Verification items for the finished model (mm, model axes). A direction names the side the tool comes from. Round coordinates to 2 decimals unless told otherwise and drop trailing zeros. Order: outer loops, then holes, each group sorted by start corner. A loop starts at its lowest first (then second) coordinate and runs counter-clockwise, first axis right, second up. Notation, with made-up numbers: (-6.75, 65.5) -> (51.25, 65.5) arc R27 ccw to (51.25, 104.5) -> close; hole circle Ø5 at (-40, 86). An arc over 180 degrees is marked (long way). Return JSON: item names as keys, results as strings. Group by question number.
1) Scan lines: L1, parallel to X at y = 0.35, z = -7; L2, parallel to X at y = 1.25, z = 11; L3, parallel to Z at x = -37, y = 2.1. Record each from-to range of solid material in increasing order.
2) Depth check by flat-ended pin: pin 1 (1.5 mm diameter, centred on x = 78, y = 1.5, fed in from -Z); pin 2 (8 mm diameter, centred on x = 4, z = -8, fed in from +Y). Enter the tip coordinate at first touch or a pass-through.
3) Section check D-D on z = 22.5. Enter the section's corners in (x, y), plus the area to 3 significant figures.
4) Section check B-B on x = -63. Enter the section's corners in (y, z).
5) Section check C-C on z = 0. State how many separate pieces and enclosed holes the cut face has, plus the area to 3 significant figures.
6) Tool access check on faces 4 (the flat face through (-18, 2, -25)), 5 (the flat face through (78, 2, -7.5)), 6 (the flat face through (-79, 2, -17.5)), 7 (the flat face through (18, 2, 25)). Record the directions out of +Z, -Z, +X, -X, +Y, -Y that give a thin tool (end or side, any length) a straight path to the whole face; none if there is none.
7) Draft check along Z on faces 1 (the flat face through (45, 2, -26)), 2 (the flat face through (-63, 2, -25)), 3 (the flat face through (-50, 2, 5.75)). Enter one of: pulls with the +Z half, pulls with the -Z half, needs draft (parallel to the pull), parting line crosses it, or undercut.
8) Section check A-A on z = 10. Enter the section's corners in (x, y).
```python
from build123d import *

# Parameters (mm, degrees)
SKETCH3_W           = 160
SKETCH3_H           = 56
BOSS_EXTRUDE1_DEPTH = 3
SKETCH4_W           = 3
SKETCH4_H           = 10
SKETCH4_W_2         = 35
SKETCH4_H_2         = 3
CUT_EXTRUDE1_DEPTH  = 85.811555816
SKETCH5_R           = 1.6
SKETCH5_R_2         = 1.5
SKETCH5_W           = 34.5
SKETCH5_H           = 24.5
SKETCH5_W_2         = 11
SKETCH5_H_2         = 30
SKETCH5_W_3         = 12.5
SKETCH5_H_3         = 11.5
CUT_EXTRUDE2_DEPTH  = 85.811555816


with BuildPart() as part:
    # Sketch3 → Boss-Extrude1 (new body)
    with BuildSketch(Plane(origin=(0, 0, 0), x_dir=(1, 0, 0), z_dir=(0, 1, 0))):
        Rectangle(SKETCH3_W, SKETCH3_H)
    extrude(amount=BOSS_EXTRUDE1_DEPTH)

    # Sketch4 → Cut-Extrude1 (cut, through all)
    with BuildSketch(Plane(origin=(0, 3, 0), x_dir=(1, 0, 0), z_dir=(0, 1, 0))):
        with Locations((-78.5, 12.5)):
            Rectangle(SKETCH4_W, SKETCH4_H)
        Polygon((-35, 28), (-35, 25), (-1.5, 25), (-1.5, 20.5), (-3, 20.5), (-3, 18), (3, 18), (3, 20.5), (1.5, 20.5), (1.5, 25), (35, 25), (35, 28), align=None)
        with Locations((-62.5, 26.5)):
            Rectangle(SKETCH4_W_2, SKETCH4_H_2)
        with Locations((62.5, 26.5)):
            Rectangle(SKETCH4_W_2, SKETCH4_H_2)
        with Locations((78.5, 12.5)):
            Rectangle(SKETCH4_W, SKETCH4_H)
        with Locations((78.5, -12.5)):
            Rectangle(SKETCH4_W, SKETCH4_H)
        with Locations((62.5, -26.5)):
            Rectangle(SKETCH4_W_2, SKETCH4_H_2)
        Polygon((35, -28), (-35, -28), (-35, -25), (-1.5, -25), (-1.5, -20.5), (-3, -20.5), (-3, -18), (3, -18), (3, -20.5), (1.5, -20.5), (1.5, -25), (35, -25), align=None)
        with Locations((-62.5, -26.5)):
            Rectangle(SKETCH4_W_2, SKETCH4_H_2)
        with Locations((-78.5, -12.5)):
            Rectangle(SKETCH4_W, SKETCH4_H)
    extrude(amount=-CUT_EXTRUDE1_DEPTH, mode=Mode.SUBTRACT)

    # Sketch5 → Cut-Extrude2 (cut, through all)
    with BuildSketch(Plane(origin=(0, 3, 0), x_dir=(1, 0, 0), z_dir=(0, 1, 0))):
        with Locations(Location((-21.5, 0, 0), (0, 0, 270))):
            Circle(SKETCH5_R)
        with Locations(Location((21.5, 0, 0), (0, 0, 90))):
            Circle(SKETCH5_R)
        with Locations(Location((-63, 0, 0), (0, 0, 270))):
            Circle(SKETCH5_R_2)
        with Locations(Location((-37, 0, 0), (0, 0, 90))):
            Circle(SKETCH5_R_2)
        Rectangle(SKETCH5_W, SKETCH5_H)
        with Locations((47.75, 0)):
            Rectangle(SKETCH5_W_2, SKETCH5_H_2)
        with Locations((-50, 0)):
            Rectangle(SKETCH5_W_3, SKETCH5_H_3)
    extrude(amount=-CUT_EXTRUDE2_DEPTH, mode=Mode.SUBTRACT)


solid = part.part
```
Check result:
{
 "1": {"L1": "-80 to -17.25, 17.25 to 42.25, 53.25 to 80", "L2": "-77 to -17.25, 17.25 to 42.25, 53.25 to 77", "L3": "-28 to -1.5, 1.5 to 28"},
 "2": {"pin 1": "z = -25", "pin 2": "through"},
 "3": {"outline": "(-80, 0) -> (-1.5, 0) -> (-1.5, 3) -> (-80, 3) -> close; (1.5, 0) -> (80, 0) -> (80, 3) -> (1.5, 3) -> close", "area": "471 mm^2"},
 "4": {"outline": "(0, -25) -> (3, -25) -> (3, -1.5) -> (0, -1.5) -> close; (0, 1.5) -> (3, 1.5) -> (3, 25) -> (0, 25) -> close"},
 "5": {"separate pieces": "8", "enclosed holes": "0", "area": "269 mm^2"},
 "6": {"face 4": "-Z, +Y, -Y", "face 5": "+X, +Y, -Y", "face 6": "-X, +Y, -Y", "face 7": "+Z, +Y, -Y"},
 "7": {"face 1": "needs draft", "face 2": "pulls with the -Z half", "face 3": "undercut"},
 "8": {"outline": "(-77, 0) -> (-17.25, 0) -> (-17.25, 3) -> (-77, 3) -> close; (17.25, 0) -> (42.25, 0) -> (42.25, 3) -> (17.25, 3) -> close; (53.25, 0) -> (77, 0) -> (77, 3) -> (53.25, 3) -> close"}
}
